Can you work these out from the model? Positions are in its coordinate system, mm. Face numbers are marked on the shaded views. A direction names the side the tool comes from. Coordinates: 2 decimals unless noted, no trailing zeros. Loops run counter-clockwise (first coordinate to the right, second up) from the corner with the lowest first, then second, coordinate; pieces in that order, holes last.
```python
from build123d import *

# Parameters (mm, degrees)
F1_DEPTH = 101.6
F3_REACH = 205.8451899427


with BuildPart() as f1:
    # F0 (on Right) → F1 (new body)
    with BuildSketch(Plane.YZ):
        with BuildLine():
            Line((-36.1766421175, -23.2471508509), (-54.3283293044, -41.0144312356))
            Line((-54.3283293044, -41.0144312356), (58.7016706956, -41.0144312356))
            Line((58.7016706956, -41.0144312356), (58.7016706956, -34.6644312356))
            Line((58.7016706956, -34.6644312356), (-13.140378273, -34.6644312356))
            Line((-13.140378273, -34.6644312356), (58.7016706956, 54.2355687644))
            Line((58.7016706956, 54.2355687644), (66.3216706956, 54.2355687644))
            Line((66.3216706956, 54.2355687644), (66.3216706956, 73.2855687644))
            Line((66.3216706956, 73.2855687644), (-13.4575252541, -25.4361495295))
            ThreePointArc((-13.4575252541, -25.4361495295), (-22.1196896865, -30.0953879884), (-31.5109779006, -27.1721532474))
            Line((-31.5109779006, -27.1721532474), (-36.1766421175, -23.2471508509))
        make_face()
        Polygon((58.7016706956, -34.6644312356), (58.7016706956, -41.0144312356), (66.3216706956, -41.0144312356), (66.3216706956, 54.2355687644), (58.7016706956, 54.2355687644), align=None)
    extrude(amount=F1_DEPTH)

    f3_end = Plane(origin=(50.8, 22.7806462113, 9.7855687644), x_dir=(0, 0.6285393611, 0.7777777778), z_dir=(0, 0.7777777778, -0.6285393611))
    # F2 (on face) → F3 (cut, up to a plane its end follows)
    with BuildSketch(Plane(origin=(0, 66.3216706956, 0), x_dir=(-1, 0, 0), z_dir=(0, 1, 0))):
        with BuildLine():
            Line((-88.9, -41.0144312356), (-12.7, -41.0144312356))
            ThreePointArc((-12.7, -41.0144312356), (-50.8, -2.9144312356), (-88.9, -41.0144312356))
        make_face()
    f3_long = extrude(amount=-F3_REACH, mode=Mode.PRIVATE)
    add(split(f3_long, bisect_by=f3_end, keep=Keep.TOP, mode=Mode.PRIVATE), mode=Mode.SUBTRACT)


solid = f1.part
```
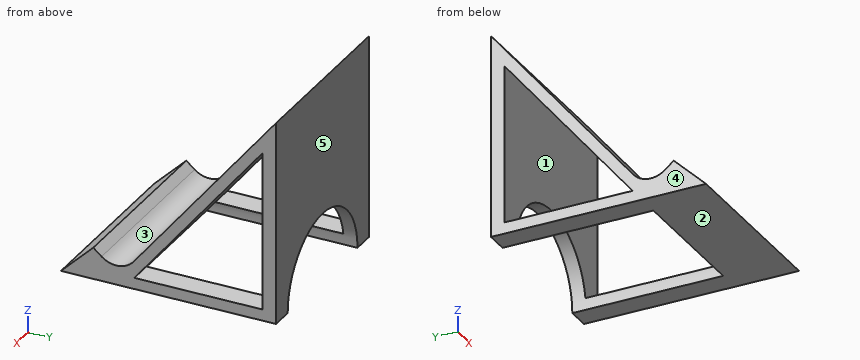
(1) I want a section at C-C on y = 6. Write out the boundary of the cut face in (x, z), then the cut area to 3 significant figures.
Check values:
outline: (0, -41.01) - (12.7, -41.01) arc R38.1 cw to (13.23, -34.66) - (0, -34.66) - close; (0, -10.98) - (101.6, -10.98) - (101.6, -1.36) - (0, -1.36) - close; (88.37, -34.66) arc R38.1 cw to (88.9, -41.01) - (101.6, -41.01) - (101.6, -34.66) - close
area: 1,140 mm2
(2) I want a section at D-D on z = 37.5. Write out the boundary of the cut face in (x, y).
Check values:
outline: (0, 37.4) - (101.6, 37.4) - (101.6, 45.18) - (0, 45.18) - close; (0, 58.7) - (101.6, 58.7) - (101.6, 66.32) - (0, 66.32) - close
(3) If we mould it in two halves opening along Y, with no side actions, what happens to the marked faces 3, 4 and 5? For each: released by +Y, released by -Y, zero draft, split by the parting line, or undercut.
Check values:
face 3: undercut
face 4: zero draft
face 5: released by +Y
(4) I'm going to push flat-ended pins straight in: pin 1 (6.5 mm diameter, centred on x = 94, y = 35, fed in from +Z); pin 2 (14.5 mm diameter, centred on x = 5.5, y = 27.5, fed in from +Z); pin 3 (5 mm diameter, centred on x = 35.5, z = -11.5, fed in from -Y). Where does each tip first touch, or does it pass through?
Check values:
pin 1: stops at z = 38.55
pin 2: stops at z = 34.22
pin 3: stops at y = -4.22
(5) If I drill on probe 1 along Z at (x, y) = (44, -22.5); probe 2 along Y at (x, z) = (61, -1); probe 3 along Y at (x, z) = (71, 33), over which ranges is the centre line in solid material (lowest first)?
Check values:
probe 1: z = -41.01 to -30.13
probe 2: y = 6.29 to 14.06, 58.7 to 66.32
probe 3: y = 33.77 to 41.54, 58.7 to 66.32
(6) Which directions (+Z, -Z, +X, -X, +Y, -Y) give clear straight access to the entire face, cutting with the end or side of a thin tool? Please do the marked faces 1 and 2.
Check values:
face 1: +X, -X
face 2: -Z, +X, -X, +Y, -Y
(7) I want a section at A-A on x = 50.8. Write out the boundary of the cut face in (y, z), then the cut area to 3 significant figures.
Check values:
outline: (-54.33, -41.01) - (-18.27, -41.01) - (58.7, 54.24) - (58.7, -2.91) - (66.32, -2.91) - (66.32, 73.29) - (-13.46, -25.44) arc R12.7 cw to (-31.51, -27.17) - (-36.18, -23.25) - close
area: 1,680 mm2
(8) I want a section at B-B on z = -7. Write out the boundary of the cut face in (x, y), then the cut area to 3 significant figures.
Check values:
outline: (0, 1.44) - (101.6, 1.44) - (101.6, 9.22) - (0, 9.22) - close; (0, 58.7) - (33.64, 58.7) - (33.64, 66.32) - (0, 66.32) - close; (67.96, 58.7) - (101.6, 58.7) - (101.6, 66.32) - (67.96, 66.32) - close
area: 1,300 mm2
